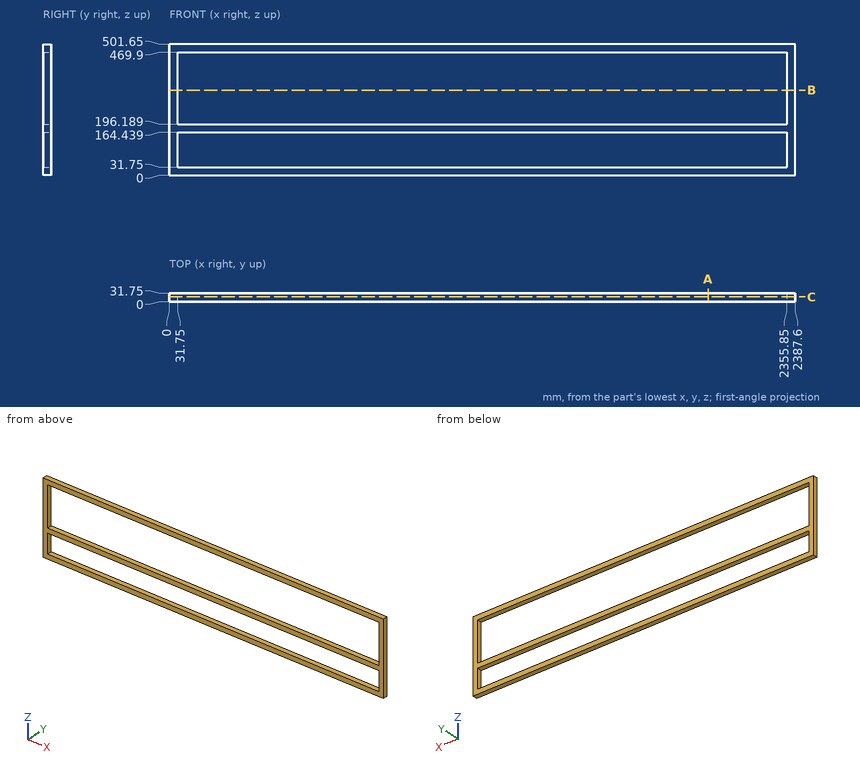
Design review of the part shown in the three views and the two pictorial views. Dimensions are in mm from the part's minimum x, y and z. Round coordinates to 2 decimals unless told otherwise and drop trailing zeros. Write each loop counter-clockwise with the first axis right and the second up, starting at its lowest first coordinate (ties: lowest second). Pieces come first, ordered by that corner, then holes.
1) Take a section at B-B on z = 326. Give the boundary of the cut face in (x, y).
Answer below:
outline: (0, 0) - (31.75, 0) - (31.75, 31.75) - (0, 31.75) - close; (2355.85, 0) - (2387.6, 0) - (2387.6, 31.75) - (2355.85, 31.75) - close
2) Take a section at C-C on y = 19. Give the boundary of the cut face in (x, z).
Answer below:
outline: (0, 0) - (2387.6, 0) - (2387.6, 501.65) - (0, 501.65) - close; hole (31.75, 31.75) - (2355.85, 31.75) - (2355.85, 164.44) - (31.75, 164.44) - close; hole (31.75, 196.19) - (2355.85, 196.19) - (2355.85, 469.9) - (31.75, 469.9) - close
3) Insertion check: pin 1 Ø3 at (x, y) = (376, 20.5) entering from -Z. The pin has a flat end and moves straight along its axis. Give the tip position at first contact, or say it passes through.
Answer below:
pin 1: stops at z = 0
4) For line 1 along Z through (x, y) = (1197.5, 26.5); line 2 along X through (y, z) = (5, 231.5), list the stretches that pass through material, from the lowest coordinate up.
Answer below:
line 1: z = 0 to 31.75, 164.44 to 196.19, 469.9 to 501.65
line 2: x = 0 to 31.75, 2355.85 to 2387.6
5) Take a section at A-A on x = 2056. Give the boundary of the cut face in (y, z), then the cut area to 3 significant figures.
Answer below:
outline: (0, 0) - (31.75, 0) - (31.75, 31.75) - (0, 31.75) - close; (0, 164.44) - (31.75, 164.44) - (31.75, 196.19) - (0, 196.19) - close; (0, 469.9) - (31.75, 469.9) - (31.75, 501.65) - (0, 501.65) - close
area: 3,020 mm2
